For this review, take the finished solid that the model builds, in its own axes (mm). Face numbers are marked on the shaded views. Coordinates: 2 decimals unless noted, no trailing zeros. Loops run counter-clockwise (first coordinate to the right, second up) from the corner with the lowest first, then second, coordinate; pieces in that order, holes last. Notation, with made-up numbers: (13, 5) - (25, 5) arc R20 cw to (25, 42) - close; hole circle Ø6 at (52, -19.75). An arc over 180 degrees is marked (long way). Use one line per item in the form item = value. Start each with the question number.
1. Add section D-D on z = -7. Give the boundary of the cut face in (x, y).
2. Draft analysis for pull direction Y (two halves, no side actions). For the marked faces 1, 2 and 3, state which applies: +Y half, -Y half, draft (parallel to the pull), parting line (faces both ways), or undercut.
3. To check wall thickness, follow probe 1 along Z at (x, y) = (4.5, 0); probe 2 along Z at (x, y) = (3.75, -0.25); probe 3 along X at (y, z) = (-8.25, 2.5). State the ranges of each line that lie inside material, in increasing order.
4. Add section C-C on x = 0.45. Give the boundary of the cut face in (y, z), and give its area (3 significant figures).
5. For pin 1 Ø1.5 at (y, z) = (-6, 3.5) entering from -X, flat-tipped, find the tip position at first contact; note if it passes through.
6. Add section A-A on z = 0. Give the boundary of the cut face in (x, y).
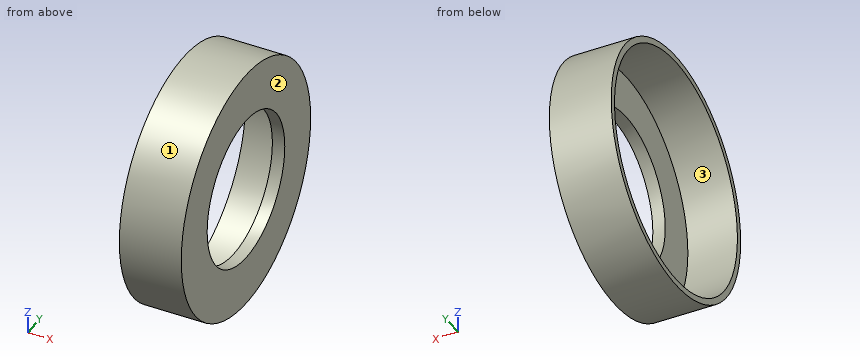
```python
from build123d import *

# Parameters (mm, degrees)
F0_R     = 10
F1_DEPTH = 5
F2_R     = 9.5
F3_DEPTH = 4
F5_D     = 12


with BuildPart() as f1:
    # F0 (on Right) → F1 (new body)
    with BuildSketch(Plane.YZ):
        Circle(F0_R)
    extrude(amount=F1_DEPTH)

    # F2 (on face) → F3 (cut)
    with BuildSketch(Plane(origin=(0, 0, 0), x_dir=(0, -1, 0), z_dir=(-1, 0, 0))):
        Circle(F2_R)
    extrude(amount=-F3_DEPTH, mode=Mode.SUBTRACT)

    # F5 (through all)
    with Locations(Plane.YZ.offset(5)):
        with Locations((0, 0)):
            Hole(F5_D / 2)


solid = f1.part
```
Conclusion:
q1.outline = (0, -7.14) - (5, -7.14) - (5, 7.14) - (0, 7.14) - (0, 6.42) - (4, 6.42) - (4, -6.42) - (0, -6.42) - close
q2.face_1 = parting line
q2.face_2 = draft
q2.face_3 = undercut
q3.probe_1 = -10 to -6, 6 to 10
q3.probe_2 = -10 to -9.5, 9.5 to 10
q3.probe_3 = 4 to 5
q4.outline = circle Ø20 at (0, 0); hole circle Ø19 at (0, 0)
q4.area = 30.6 mm^2
q5.pin_1 = 4
q6.outline = (0, -10) - (5, -10) - (5, -6) - (4, -6) - (4, -9.5) - (0, -9.5) - close; (0, 9.5) - (4, 9.5) - (4, 6) - (5, 6) - (5, 10) - (0, 10) - close
